For this review, use the dimensioned drawing (mm, ordinates from the lowest corner) and the shaded views. Round coordinates to 2 decimals unless told otherwise and drop trailing zeros. Order: outer loops, then holes, each group sorted by start corner. A loop starts at its lowest first (then second) coordinate and runs counter-clockwise, first axis right, second up. Notation, with made-up numbers: M 5.5,47 L 52.5,47 A25 ccw 52.5,67 Z; hole C -35.5,36 d5. An arc over 180 degrees is marked long. Put each result on its own line as item: value.
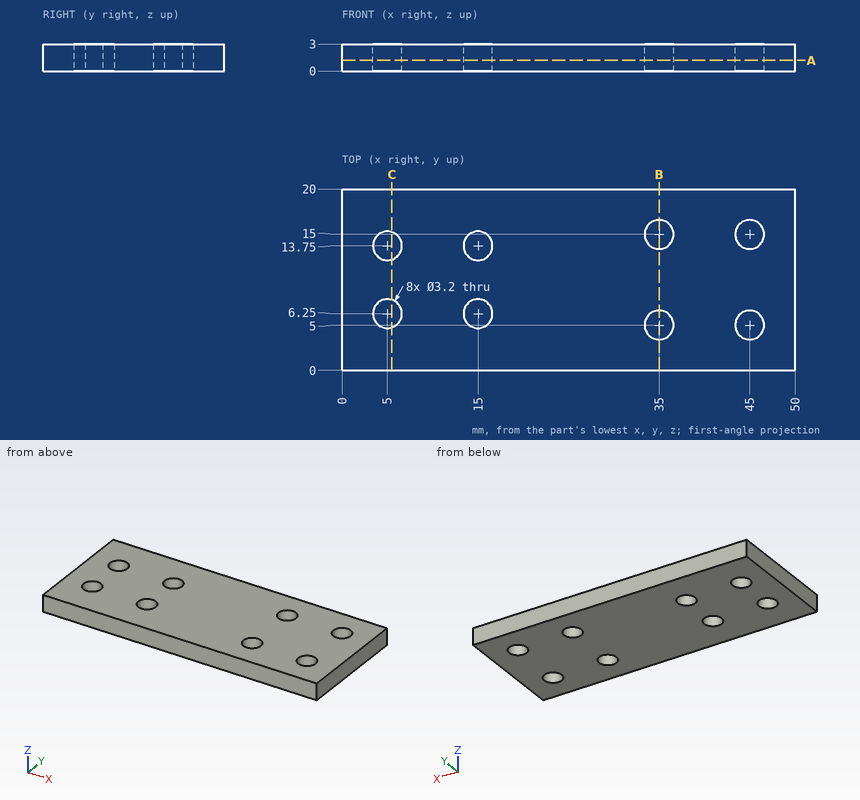
(1) Add section C-C on x = 5.5. Give the boundary of the cut face in (y, z), then the cut area to 3 significant figures.
A:
outline: M 0,0 L 4.73,0 L 4.73,3 L 0,3 Z; M 7.77,0 L 12.23,0 L 12.23,3 L 7.77,3 Z; M 15.27,0 L 20,0 L 20,3 L 15.27,3 Z
area: 41.8 mm2
(2) Add section B-B on x = 35. Give the boundary of the cut face in (y, z).
A:
outline: M 0,0 L 3.4,0 L 3.4,3 L 0,3 Z; M 6.6,0 L 13.4,0 L 13.4,3 L 6.6,3 Z; M 16.6,0 L 20,0 L 20,3 L 16.6,3 Z
(3) Add section A-A on z = 1.2. State how many separate pieces and enclosed holes the cut face has, then the cut area to 3 significant figures.
A:
separate pieces: 1
enclosed holes: 8
area: 936 mm2
(4) To check wall thickness, follow L1, parallel to Y at x = 45, z = 1.35; L2, parallel to X at y = 4, z = 2.8; L3, parallel to X at y = 14, z = 0.3. State the ranges of each line that lie inside material, in increasing order.
A:
L1: y = 0 to 3.4, 6.6 to 13.4, 16.6 to 20
L2: x = 0 to 33.75, 36.25 to 43.75, 46.25 to 50
L3: x = 0 to 3.42, 6.58 to 13.42, 16.58 to 33.75, 36.25 to 43.75, 46.25 to 50
(5) Insertion check: pin 1 Ø5 at (x, y) = (33.5, 8.5) entering from -Z. The pin has a flat end and moves straight along its axis. Give the tip position at first contact, or say it passes through.
A:
pin 1: stops at z = 0
